from build123d import *

# Parameters (mm, degrees)
REVOLUTION003_ANGLE       = -180
PAD019_DEPTH              = 0.4
BODY018_PLACEMENT_ANGLE   = 180
PAD018_DEPTH              = 2.4
FUSION004_PLACEMENT_ANGLE = 10


with BuildPart() as light003:
    # Sketch030 (on Face1 of ShapeBinder007) → Revolution003 (revolve)
    with BuildSketch(Plane.XY.offset(2.4)):
        with BuildLine():
            ThreePointArc((-2.75, 0), (0, -2.75), (2.75, 0))
            Line((-2.75, 0), (2.75, 0))
        make_face()
    revolve(axis=Axis((-2.75, 0, 2.4), (1, 0, 0)), revolution_arc=REVOLUTION003_ANGLE)


with BuildPart() as body018:
    # Sketch031 (on Face1 of ShapeBinder008) → Pad019 (new body)
    with BuildSketch(Plane(origin=(0, 0, 0), x_dir=(1, 0, 0), z_dir=(0, 0, -1))):
        with BuildLine():
            Line((3.65, 1.5), (6.65, 1.5))
            Line((6.65, 1.5), (6.65, 2))
            Line((6.65, 2), (8.65, 2))
            Line((8.65, 2), (8.65, 0.2))
            Line((8.65, 0.2), (6.65, 0.2))
            Line((6.65, 0.2), (6.65, 0.7))
            Line((6.65, 0.7), (4.45, 0.7))
            Line((4.45, 0.7), (4.45, -0.2))
            ThreePointArc((4.45, -0.2), (3.8, -0.85), (4.45, -1.5))
            Line((4.45, -1.5), (-6.65, -1.5))
            Line((-6.65, -1.5), (-6.65, -1.85))
            Line((-6.65, -1.85), (-8.65, -1.85))
            Line((-8.65, -1.85), (-8.65, -0.25))
            Line((-8.65, -0.25), (-6.65, -0.25))
            Line((-6.65, -0.25), (-6.65, -0.6))
            Line((-6.65, -0.6), (-4.95, -0.6))
            Line((-4.95, -0.6), (-4.95, 1.5))
            Line((-4.95, 1.5), (3.65, 1.5))
        make_face()
    extrude(amount=-PAD019_DEPTH)


with BuildPart() as body018_1:
    # Body018 placement: moved
    add(body018.part.moved(Location((0, 0, 1.4))).rotate(Axis((0, 0, 1.4), (1, 0, 0)), BODY018_PLACEMENT_ANGLE))


with BuildPart() as led4:
    # Sketch029 → Pad018 (new body)
    with BuildSketch(Plane.XY):
        with BuildLine():
            Line((-3.65, 1.75), (-3.65, -1.75))
            ThreePointArc((-3.65, -1.75), (0, -4), (3.65, -1.75))
            Line((3.65, 1.75), (3.65, -1.75))
            ThreePointArc((3.65, 1.75), (0, 4), (-3.65, 1.75))
        make_face()
    extrude(amount=PAD018_DEPTH)

    # Fusion004: union light003, Body018
    add(light003.part)
    add(body018_1.part)


with BuildPart() as led4_1:
    # Fusion004 placement: moved
    add(led4.part.moved(Location((27, -36.5, -2.8))).rotate(Axis((27, -36.5, -2.8), (0, 0, 1)), FUSION004_PLACEMENT_ANGLE))


solid = led4_1.part
Design review of the part built by this model. Coordinates are the model's own, in mm. A direction names the side the tool comes from. Coordinates: 2 decimals unless noted, no trailing zeros. Loops run counter-clockwise (first coordinate to the right, second up) from the corner with the lowest first, then second, coordinate; pieces in that order, holes last. Notation, with made-up numbers: (87, 51.5) -> (112, 51.5) arc R28 ccw to (112, 78.5) -> close; hole circle Ø7 at (34, -8). An arc over 180 degrees is marked (long way). Use a Markdown table: item, result. Add a question column.
Item 1: We need section C-C, the plane y = -36.5. Write out the cut boundary in (x, z), and give its area (3 significant figures).
Item 2: We need section A-A, the plane x = 25. Write out the cut boundary in (y, z).
Item 3: We need section B-B, the plane z = -2.05. Write out the cut boundary in (x, y), and give its area (3 significant figures).
Item 4: Wall thickness on L1, parallel to Z at x = 29.5, y = -39; L2, parallel to Y at x = 29.5, z = -1.25; L3, parallel to X at y = -35.5, z = 0.6: over which ranges is each line inside the solid? List them lowest first. Write a range as from..to.
Item 5: We need section D-D, the plane z = 0.4. Write out the cut boundary in (x, y), and give its area (3 significant figures).
Item 6: Machinability: for faces 1 (the flat face through (21.7, -38.3, -1.4)), 2 (the flat face through (21.7, -38.3, -1.8)), 3 (the flat face through (27, -36, -2.8)), 4 (the flat face through (24, -35, -0.4)), which of the approach directions +Z, -Z, +X, -X, +Y, -Y give a long, thin tool a straight path to every point of the face, cutting with its end or side? Answer none if there is none.
Item 7: Clearance check with flat-ended pins moving along their axes: P1, Ø3.5, axis at x = 20, y = -38.5, coming from the +Z side; P2, Ø4.5, axis at x = 21.5, y = -37.5, coming from the -Z side; P3, Ø1.5, axis at x = 25, z = -1, coming from the +Y side; P4, Ø2.5, axis at x = 29, y = -38, coming from the +Z side. State where each tip first meets the part, or that it passes through.
Numbers:
| question | item | result |
|---|---|---|
| 1 | outline | (21.97, -1.8) -> (23.29, -1.8) -> (23.29, -2.8) -> (30.71, -2.8) -> (30.71, -1.8) -> (30.88, -1.8) -> (30.88, -1.4) -> (30.71, -1.4) -> (30.71, -0.4) -> (29.75, -0.4) arc R2.75 ccw to (24.25, -0.4) -> (23.29, -0.4) -> (23.29, -1.4) -> (21.97, -1.4) -> close |
| 1 | area | 30.3 mm^2 |
| 2 | outline | (-39.99, -2.8) -> (-33.03, -2.8) -> (-33.03, -0.4) -> (-34.61, -0.4) arc R1.89 ccw to (-38.39, -0.4) -> (-39.99, -0.4) -> close |
| 3 | outline | (23.1, -35.41) -> (23.71, -38.86) arc R4.09 ccw to (30.9, -37.59) -> (30.29, -34.14) arc R4.09 ccw to start |
| 3 | area | 49.0 mm^2 |
| 4 | L1 | z = -2.8..-0.4 |
| 4 | L2 | y = -39.64..-33.34 |
| 4 | L3 | x = 24.64..29.36 |
| 5 | outline | circle Ø5.26 at (27, -36.5) |
| 5 | area | 21.7 mm^2 |
| 6 | face 1 | +Z, -X, -Y |
| 6 | face 2 | -Z, -X, -Y |
| 6 | face 3 | -Z, +X, -X, +Y, -Y |
| 6 | face 4 | +Z |
| 7 | P1 | stops at z = -1.4 |
| 7 | P2 | stops at z = -2.8 |
| 7 | P3 | stops at y = -32.7 |
| 7 | P4 | stops at z = 2.05 |
